Source: three-view drawing plus pictorial views. Frame: mm from the lowest corner of the part. A direction names the side the tool comes from. Give positions to 0.01 mm unless a question says otherwise; leave off trailing zeros. Write each loop counter-clockwise with the first axis right and the second up, starting at its lowest first coordinate (ties: lowest second). Pieces come first, ordered by that corner, then holes. Notation, with made-up numbers: (35.25, -8.5) -> (94.25, -8.5) arc R32 ccw to (94.25, 18.5) -> close; hole circle Ø5 at (67.5, 72). An arc over 180 degrees is marked (long way). Write item = value, one per line.
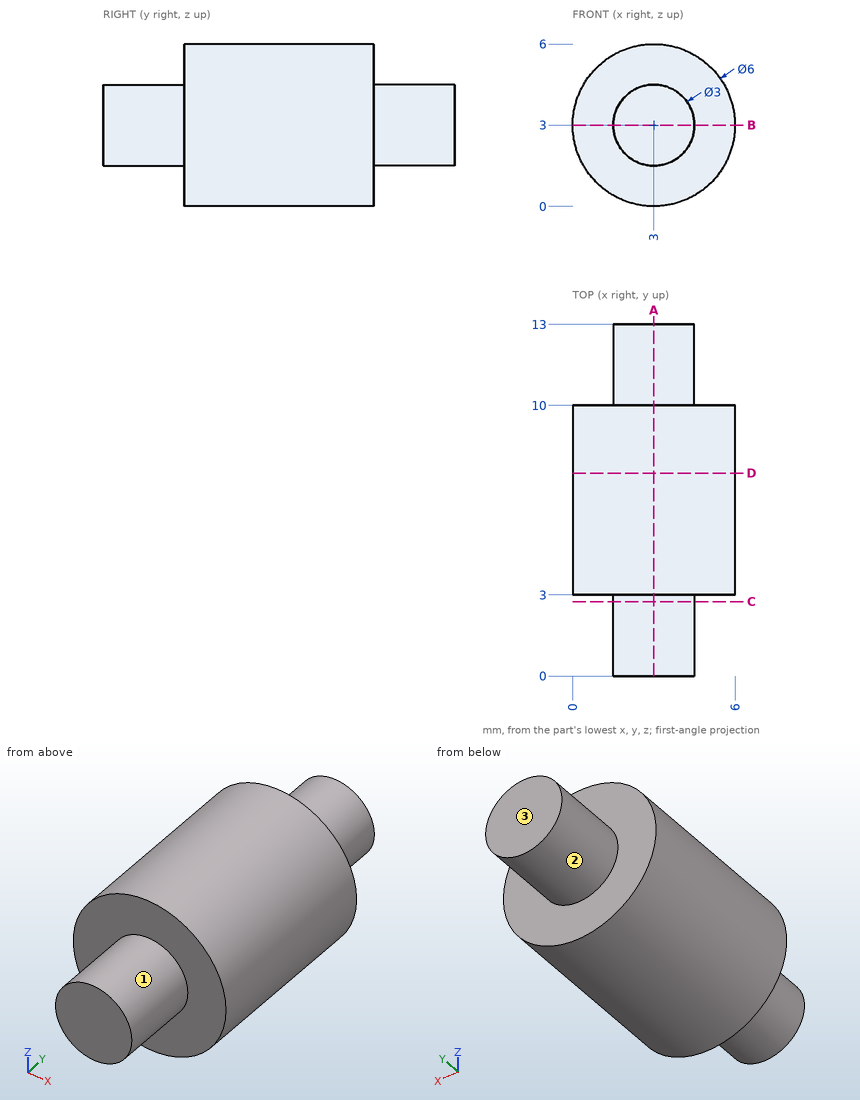
1) Cut plane C-C (y = 2.75). Return the cut outline in (x, z), then the cut area to 3 significant figures.
Computed:
outline = circle Ø3 at (3, 3)
area = 7.07 mm²
2) Access query for the marked faces 1, 2 and 3. Directions: +Z, -Z, +X, -X, +Y, -Y. A direction counts if a zero-diameter tool reaches every point of the face in a straight line with its end or side. Return the directions, or none.
Computed:
face_1 = -Y
face_2 = +Y
face_3 = +Z, -Z, +X, -X, +Y
3) Material intervals for L1, parallel to Z at x = 3.1, y = 3.5; L2, parallel to Y at x = 0.8, z = 4; L3, parallel to Z at x = 1.9, y = 10.5, sorted ascending.
Computed:
L1 = 0 to 6
L2 = 3 to 10
L3 = 1.98 to 4.02
4) Cut plane D-D (y = 7.5). Return the cut outline in (x, z), then the cut area to 3 significant figures.
Computed:
outline = circle Ø6 at (3, 3)
area = 28.3 mm²
5) Cut plane A-A (x = 3). Return the cut outline in (y, z), then the cut area to 3 significant figures.
Computed:
outline = (0, 1.5) -> (3, 1.5) -> (3, 0) -> (10, 0) -> (10, 1.5) -> (13, 1.5) -> (13, 4.5) -> (10, 4.5) -> (10, 6) -> (3, 6) -> (3, 4.5) -> (0, 4.5) -> close
area = 60.0 mm²
6) Contact query for flat-ended pins moving along their axis: pin 1 (1.5 mm diameter, centred on y = 3.5, z = 5.5, fed in from +X); pin 2 (1 mm diameter, centred on y = 11.5, z = 0.5, fed in from +X); pin 3 (1.5 mm diameter, centred on y = 11, z = 4, fed in from -X). Output: stop coordinate, or through.
Computed:
pin_1 = 5.44
pin_2 = through
pin_3 = 1.52
7) Cut plane B-B (z = 3). Return the cut outline in (x, y).
Computed:
outline = (0, 3) -> (1.5, 3) -> (1.5, 0) -> (4.5, 0) -> (4.5, 3) -> (6, 3) -> (6, 10) -> (4.5, 10) -> (4.5, 13) -> (1.5, 13) -> (1.5, 10) -> (0, 10) -> close
